Work out the finished part from the listing and answer in its coordinate system (mm). A direction names the side the tool comes from. Give positions to 0.01 mm unless a question says otherwise; leave off trailing zeros. Loops run counter-clockwise (first coordinate to the right, second up) from the corner with the lowest first, then second, coordinate; pieces in that order, holes last. Notation, with made-up numbers: M -24,48.5 L -9,48.5 A27 cw -9,76.5 Z; hole C -6.5,87 d9. An arc over 180 degrees is marked long. Write item = value, one per line. Start each with the question number.
1. Section A-A on z = 9.75 is taken. Determine the outline of the cut face in (x, y).
2. The mould has two halves that part along X. Classify faces 1 (the face through (19.622, 9, 5)), 2 (the face through (-4.234, -11, 9)), 3 (the face through (20, -5, 12.382)): released by +X, released by -X, zero draft, split by the parting line, or undercut.
3. Flat-ended cylindrical pins translate along their axes: pin 1 Ø4 at (x, z) = (10, 7) entering from -Y; pin 2 Ø6 at (x, y) = (-10, -3.5) entering from +Z; pin 3 Ø4.5 at (y, z) = (7.5, 5.5) entering from +X. Find the tip coordinate at first contact, or state that the pin passes through.
4. Consider L1, parallel to Y at x = -17, z = 9.5; L2, parallel to X at y = -4.75, z = 10.25; L3, parallel to Y at x = 2, z = 9.75. Determine where each line is inside the solid, lowest interval first. Write a range as [from, to].
5. Section D-D on x = -17 is taken. Determine the outline of the cut face in (y, z), plus the area to 3 significant figures.
6. Section B-B on y = -1.5 is taken. Determine the outline of the cut face in (x, z).
7. Section C-C on z = 1 is taken. Determine the outline of the cut face in (x, y).
8. For faces 4 (the face through (-14.928, -6, 9)), 5 (the face through (-19.26, 2.35, 8.63)), 6 (the face through (21.97, -4.59, 9.05)), determine the directions among +Z, -Z, +X, -X, +Y, -Y from which every point of the face is accessible in a straight line to the end or side of a thin tool.
```python
from build123d import *

# Parameters (mm, degrees)
F0_W     = 39.243
F0_H     = 25.4254
F1_DEPTH = 4.7625
F2_W     = 4.69392
F2_H     = 15.4432
F2_W_2   = 10.2489
F2_H_2   = 3.1115
F2_W_3   = 39.243
F2_H_3   = 4.7625
F3_DEPTH = 7.62
F5_DEPTH = 4.7625
F7_D     = 5.7658
F7_DEPTH = 4.7625
F7_TIP   = 1.7322210786
F8_R     = 1.27


# Not quite as in the source:
# - a length typed as a fraction of an inch, garbled in the dataset ("3 / 203.2 mm" for 3/8 in), is restored


with BuildPart() as f1:
    # F0 (on Top) → F1 (new body)
    with BuildSketch(Plane.XY):
        Rectangle(F0_W, F0_H)
    extrude(amount=F1_DEPTH)

    # F2 (on face) → F3 (join)
    with BuildSketch(Plane.XY.offset(4.7625)):
        with Locations((-17.27454, -4.9911)):
            Rectangle(F2_W, F2_H)
        with Locations((17.27454, -4.9911)):
            Rectangle(F2_W, F2_H)
        with Locations((0.89027, -11.15695)):
            Rectangle(F2_W_2, F2_H_2)
        with Locations((0, 10.33145)):
            Rectangle(F2_W_3, F2_H_3)
    extrude(amount=F3_DEPTH)

    # F4 (on face) → F5 (join)
    with BuildSketch(Plane.YZ.offset(19.6215)):
        Polygon((2.7305, 4.7625), (2.7305, 12.3825), (-12.7127, 12.3825), (-12.7127, 0), (2.7305, 0), align=None)
    extrude(amount=F5_DEPTH)

    # F7
    with Locations(Plane.YZ.offset(24.384)):
        with Locations((-4.9657, 6.19125)):
            Hole(F7_D / 2, depth=F7_DEPTH)
            with Locations((0, 0, -(F7_DEPTH + F7_TIP / 2))):  # 118° drill point
                Cone(0, F7_D / 2, F7_TIP, mode=Mode.SUBTRACT)

    # F8
    f8_edges = [f1.edges().sort_by_distance(p)[0] for p in [
        (-14.92758, 2.7305, 8.5725),
        (14.92758, 2.7305, 8.5725),
        (-19.6215, -12.7127, 6.19125),
        (24.384, -12.7127, 6.19125),
        (24.384, 2.7305, 6.19125),
        (19.6215, 12.7127, 6.19125),
        (-19.6215, 12.7127, 6.19125),
        (-19.6215, 2.7305, 8.5725),
    ]]
    fillet(f8_edges, radius=F8_R)


solid = f1.part
```
Verdict:
q1.outline = M -19.62,-11.44 A1.27 ccw -18.35,-12.71 L -14.93,-12.71 L -14.93,1.46 A1.27 ccw -16.2,2.73 L -18.35,2.73 A1.27 ccw -19.62,1.46 Z; M -19.62,7.95 L 19.62,7.95 L 19.62,11.44 A1.27 ccw 18.35,12.71 L -18.35,12.71 A1.27 ccw -19.62,11.44 Z; M -4.23,-12.71 L 6.01,-12.71 L 6.01,-9.6 L -4.23,-9.6 Z; M 14.93,-12.71 L 23.11,-12.71 A1.27 ccw 24.38,-11.44 L 24.38,1.46 A1.27 ccw 23.11,2.73 L 16.2,2.73 A1.27 ccw 14.93,1.46 Z
q2.face_1 = released by +X
q2.face_2 = undercut
q2.face_3 = zero draft
q3.pin_1 = 7.95
q3.pin_2 = 4.76
q3.pin_3 = 19.62
q4.L1 = [-12.71, 2.73], [7.95, 12.71]
q4.L2 = [-19.62, -14.93], [14.93, 24.38]
q4.L3 = [-12.71, -9.6], [7.95, 12.71]
q5.outline = M -12.71,0 L 12.71,0 L 12.71,12.38 L 7.95,12.38 L 7.95,4.76 L 2.73,4.76 L 2.73,12.38 L -12.71,12.38 Z
q5.area = 275 mm2
q6.outline = M -19.62,0 L 24.38,0 L 24.38,12.38 L 14.93,12.38 L 14.93,4.76 L -14.93,4.76 L -14.93,12.38 L -19.62,12.38 Z
q7.outline = M -19.62,-11.44 A1.27 ccw -18.35,-12.71 L 23.11,-12.71 A1.27 ccw 24.38,-11.44 L 24.38,1.46 A1.27 ccw 23.11,2.73 L 19.62,2.73 L 19.62,11.44 A1.27 ccw 18.35,12.71 L -18.35,12.71 A1.27 ccw -19.62,11.44 Z
q8.face_4 = +Z, -Y
q8.face_5 = +Z, -X
q8.face_6 = +X
